Answer from the drawing. Dimensions are ordinates in mm from the lowest x, y and z of the part. Give positions to 0.01 mm unless a question says otherwise; leave off trailing zeros. Write each loop counter-clockwise with the first axis right and the second up, starting at its lowest first coordinate (ties: lowest second). Pieces come first, ordered by that corner, then holes. Notation, with made-up numbers: M 79,-26 L 93,-26 A16 ccw 93,-16 Z; hole C 1,-37.75 d3. An arc over 180 degrees is marked long. Write each question's results on one line, items separated by ' | '. Start each with the question number.
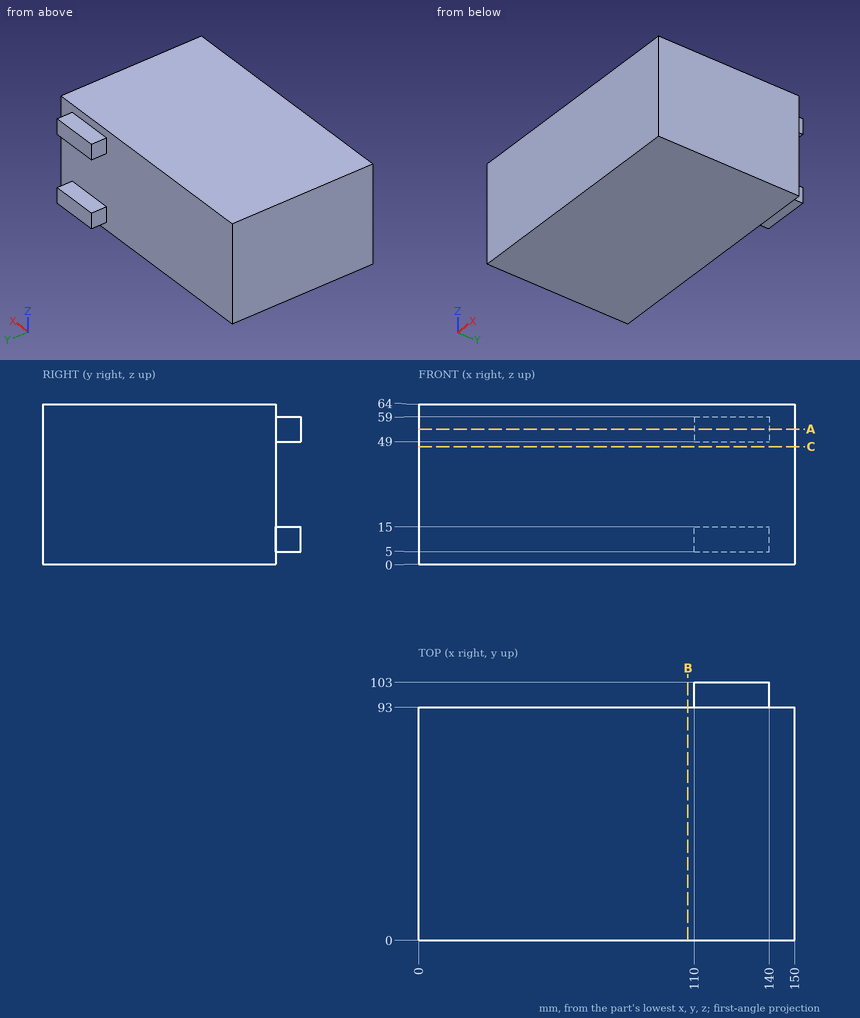
Item 1: Section A-A, the plane z = 54 is taken. Determine the outline of the cut face in (x, y).
Item 2: Straight lines are drawn through the part: line 1 (Y direction, x = 48.5, z = 23); line 2 (Z direction, x = 138.5, y = 93.5). For each, find the intervals that lie inside material, in ascending order.
Item 3: Section C-C, the plane z = 47 is taken. Determine the outline of the cut face in (x, y), then the cut area to 4 significant figures.
Item 4: Given P1, Ø1.5, axis at x = 108.5, z = 7.5, coming from the +Y side; P2, Ø5, axis at y = 98.5, z = 9, coming from the +X side; P3, Ø5, axis at y = 98.5, z = 11.5, coming from the -X side, each flat-ended and moving along its own axis, determine where each tip first touches the part or whether it passes through.
Item 5: Section B-B, the plane x = 107.5 is taken. Determine the outline of the cut face in (y, z), then the cut area to 3 significant figures.
Worked out:
1) outline: M 0,0 L 150,0 L 150,93 L 140,93 L 140,103 L 110,103 L 110,93 L 0,93 Z
2) line 1: y = 0 to 93 | line 2: z = 5 to 15, 49 to 59
3) outline: M 0,0 L 150,0 L 150,93 L 0,93 Z | area: 13,950 mm²
4) P1: stops at y = 93 | P2: stops at x = 140 | P3: stops at x = 110
5) outline: M 0,0 L 93,0 L 93,64 L 0,64 Z | area: 5,950 mm²
